Build history of the part. All positions in model axes, mm. Give positions to 0.01 mm unless a question says otherwise; leave off trailing zeros. Loops run counter-clockwise (first coordinate to the right, second up) from the corner with the lowest first, then second, coordinate; pieces in that order, holes last. Notation, with made-up numbers: (66.5, 61.5) - (79.5, 61.5) arc R12 ccw to (79.5, 71.5) - close; hole circle Ø2 at (-30, 72.5). An arc over 180 degrees is marked (long way). Return JSON: item names as keys, results as strings. Group by question number.
1) Drop a flat-ended pin along its axis: pin 1 (1 mm diameter, centred on y = 0.5, z = -23.5, fed in from -X). Give the stop position or say it passes through.
2) Slice it at A-A (z = -27.5). List the corners of the cut face in (x, y), and give its area (3 significant figures).
3) Slice it at C-C (z = 14). List the corners of the cut face in (x, y).
4) Slice it at B-B (y = 1.65). Count the separate pieces of the cut face and the enclosed holes in it, and give its area (3 significant figures).
5) Drill centre lines: probe 1 along X at (y, z) = (2.15, 0); probe 2 along X at (y, z) = (0.45, -65); probe 3 along Z at (x, y) = (-33.5, 2.05). Where is each one in solid material? Low to high. Write a range as from..to.
```python
from build123d import *

# Parameters (mm, degrees)
IZIM1_R                     = 100
IZIM1_R_2                   = 71.5
Y_KSEKLIK_EKSTR_ZYON1_DEPTH = 3
IZIM2_R                     = 1.9
KES_EKSTR_ZYON1_DEPTH       = 142.453172464
DAIRESEL_KAPLAMA1_COUNT     = 6


with BuildPart() as part:
    # Çizim1 → Yükseklik-Ekstrüzyon1 (new body)
    with BuildSketch(Plane(origin=(0, 0, 0), x_dir=(1, 0, 0), z_dir=(0, 1, 0))):
        with Locations(Location((0, 0, 0), (0, 0, 270))):
            Circle(IZIM1_R)
        with Locations(Location((0, 0, 0), (0, 0, 270))):
            Circle(IZIM1_R_2, mode=Mode.SUBTRACT)
    extrude(amount=Y_KSEKLIK_EKSTR_ZYON1_DEPTH)

    # Çizim2 → Kes-Ekstrüzyon1 (cut, symmetric)
    with BuildSketch(Plane(origin=(0, 3, 0), x_dir=(1, 0, 0), z_dir=(0, 1, 0))):
        with Locations(Location((-95, 0, 0), (0, 0, 270))):
            Circle(IZIM2_R)
        with Locations(Location((-75, 0, 0), (0, 0, 270))):
            Circle(IZIM2_R)
    kes_ekstr_zyon1 = extrude(amount=KES_EKSTR_ZYON1_DEPTH, both=True, mode=Mode.SUBTRACT)

    # Dairesel Kaplama1: Kes-Ekstrüzyon1 ×6 about axis
    dairesel_kaplama1_axis = Axis((0, 0, 0), (0, 1, 0))
    for i in range(1, DAIRESEL_KAPLAMA1_COUNT):
        add(kes_ekstr_zyon1.rotate(dairesel_kaplama1_axis, i * 360 / DAIRESEL_KAPLAMA1_COUNT), mode=Mode.SUBTRACT)


solid = part.part
```
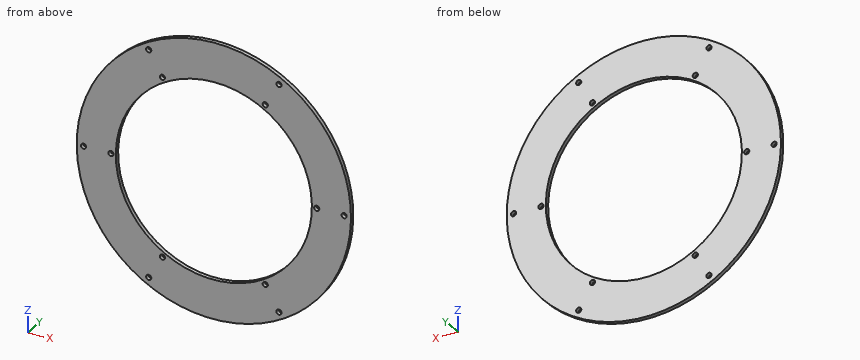
Results:
{
 "1": {"pin 1": "x = -97.32"},
 "2": {"outline": "(-96.14, 0) - (-66, 0) - (-66, 3) - (-96.14, 3) - close; (66, 0) - (96.14, 0) - (96.14, 3) - (66, 3) - close", "area": "181 mm2"},
 "3": {"outline": "(-99.02, 0) - (-70.12, 0) - (-70.12, 3) - (-99.02, 3) - close; (70.12, 0) - (99.02, 0) - (99.02, 3) - (70.12, 3) - close"},
 "4": {"separate pieces": "1", "enclosed holes": "13", "area": "15,200 mm2"},
 "5": {"probe 1": "-100..-96.9, -93.1..-76.9, -73.1..-71.5, 71.5..73.1, 76.9..93.1, 96.9..100", "probe 2": "-75.99..-39.4, -35.6..-29.79, 29.79..35.6, 39.4..75.99", "probe 3": "-94.22..-63.17, 63.17..94.22"}
}
